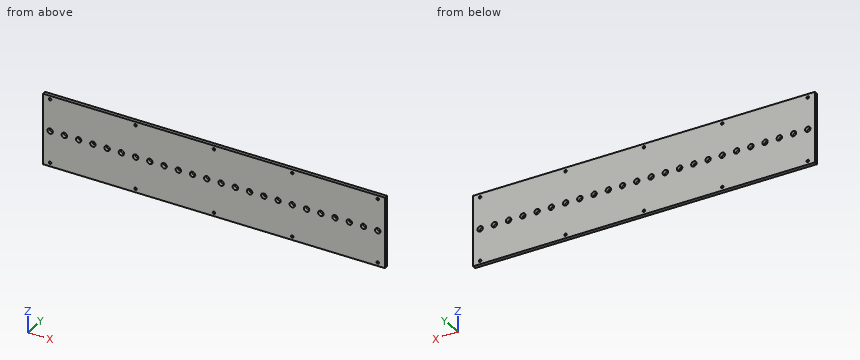
from build123d import *

# Parameters (mm, degrees)
SKETCH2_W           = 609.6
SKETCH2_H           = 127
SKETCH2_R           = 4.826
BOSS_EXTRUDE1_DEPTH = 6.35
SKETCH3_R           = 2.1828125
CUT_EXTRUDE1_DEPTH  = 6.35


with BuildPart() as part:
    # Sketch2 → Boss-Extrude1 (new body)
    with BuildSketch(Plane(origin=(0, 0, 0), x_dir=(1, 0, 0), z_dir=(0, 1, 0))):
        with Locations((304.8, 63.5)):
            Rectangle(SKETCH2_W, SKETCH2_H)
        with Locations(Location((12.7, 63.5, 0), (0, 0, 270))):
            Circle(SKETCH2_R, mode=Mode.SUBTRACT)
        with Locations(Location((38.1, 63.5, 0), (0, 0, 270))):
            Circle(SKETCH2_R, mode=Mode.SUBTRACT)
        with Locations(Location((63.5, 63.5, 0), (0, 0, 270))):
            Circle(SKETCH2_R, mode=Mode.SUBTRACT)
        with Locations(Location((88.9, 63.5, 0), (0, 0, 270))):
            Circle(SKETCH2_R, mode=Mode.SUBTRACT)
        with Locations(Location((114.3, 63.5, 0), (0, 0, 270))):
            Circle(SKETCH2_R, mode=Mode.SUBTRACT)
        with Locations(Location((139.7, 63.5, 0), (0, 0, 270))):
            Circle(SKETCH2_R, mode=Mode.SUBTRACT)
        with Locations(Location((165.1, 63.5, 0), (0, 0, 270))):
            Circle(SKETCH2_R, mode=Mode.SUBTRACT)
        with Locations(Location((190.5, 63.5, 0), (0, 0, 270))):
            Circle(SKETCH2_R, mode=Mode.SUBTRACT)
        with Locations(Location((215.9, 63.5, 0), (0, 0, 270))):
            Circle(SKETCH2_R, mode=Mode.SUBTRACT)
        with Locations(Location((241.3, 63.5, 0), (0, 0, 270))):
            Circle(SKETCH2_R, mode=Mode.SUBTRACT)
        with Locations(Location((266.7, 63.5, 0), (0, 0, 270))):
            Circle(SKETCH2_R, mode=Mode.SUBTRACT)
        with Locations(Location((292.1, 63.5, 0), (0, 0, 270))):
            Circle(SKETCH2_R, mode=Mode.SUBTRACT)
        with Locations(Location((317.5, 63.5, 0), (0, 0, 270))):
            Circle(SKETCH2_R, mode=Mode.SUBTRACT)
        with Locations(Location((342.9, 63.5, 0), (0, 0, 270))):
            Circle(SKETCH2_R, mode=Mode.SUBTRACT)
        with Locations(Location((368.3, 63.5, 0), (0, 0, 270))):
            Circle(SKETCH2_R, mode=Mode.SUBTRACT)
        with Locations(Location((393.7, 63.5, 0), (0, 0, 270))):
            Circle(SKETCH2_R, mode=Mode.SUBTRACT)
        with Locations(Location((419.1, 63.5, 0), (0, 0, 270))):
            Circle(SKETCH2_R, mode=Mode.SUBTRACT)
        with Locations(Location((444.5, 63.5, 0), (0, 0, 270))):
            Circle(SKETCH2_R, mode=Mode.SUBTRACT)
        with Locations(Location((469.9, 63.5, 0), (0, 0, 270))):
            Circle(SKETCH2_R, mode=Mode.SUBTRACT)
        with Locations(Location((495.3, 63.5, 0), (0, 0, 270))):
            Circle(SKETCH2_R, mode=Mode.SUBTRACT)
        with Locations(Location((520.7, 63.5, 0), (0, 0, 270))):
            Circle(SKETCH2_R, mode=Mode.SUBTRACT)
        with Locations(Location((546.1, 63.5, 0), (0, 0, 270))):
            Circle(SKETCH2_R, mode=Mode.SUBTRACT)
        with Locations(Location((571.5, 63.5, 0), (0, 0, 270))):
            Circle(SKETCH2_R, mode=Mode.SUBTRACT)
        with Locations(Location((596.9, 63.5, 0), (0, 0, 270))):
            Circle(SKETCH2_R, mode=Mode.SUBTRACT)
    extrude(amount=BOSS_EXTRUDE1_DEPTH)

    # Sketch3 → Cut-Extrude1 (cut)
    with BuildSketch(Plane(origin=(0, 6.35, 0), x_dir=(1, 0, 0), z_dir=(0, 1, 0))):
        with Locations(Location((12.7, 120.65, 0), (0, 0, 270))):
            Circle(SKETCH3_R)
        with Locations(Location((165.1, 120.65, 0), (0, 0, 270))):
            Circle(SKETCH3_R)
        with Locations(Location((304.8, 120.65, 0), (0, 0, 270))):
            Circle(SKETCH3_R)
        with Locations(Location((444.5, 120.65, 0), (0, 0, 270))):
            Circle(SKETCH3_R)
        with Locations(Location((596.9, 120.65, 0), (0, 0, 270))):
            Circle(SKETCH3_R)
        with Locations(Location((596.9, 6.35, 0), (0, 0, 270))):
            Circle(SKETCH3_R)
        with Locations(Location((444.5, 6.35, 0), (0, 0, 270))):
            Circle(SKETCH3_R)
        with Locations(Location((304.8, 6.35, 0), (0, 0, 270))):
            Circle(SKETCH3_R)
        with Locations(Location((165.1, 6.35, 0), (0, 0, 270))):
            Circle(SKETCH3_R)
        with Locations(Location((12.7, 6.35, 0), (0, 0, 270))):
            Circle(SKETCH3_R)
    extrude(amount=-CUT_EXTRUDE1_DEPTH, mode=Mode.SUBTRACT)


solid = part.part
Part model, mm, in its own coordinate system. Give positions to 0.01 mm unless a question says otherwise; leave off trailing zeros. Write each question's results on one line, items separated by ' | '. Start each with the question number.
Q1. Wall check: L1, parallel to Z at x = 445, y = 3.75; L2, parallel to X at y = 4.75, z = -6.35; L3, parallel to Z at x = 39, y = 5.5. Give the ranges that are in metal, low to high.
Q2. Band-saw the part on A-A on y = 1.5. Count the separate pieces of the cut face and the enclosed holes in it, plus the area to 3 significant figures.
Q3. Pin check, flat tip, straight feed: P1, Ø7.5, axis at x = 190.5, z = -63.5, coming from the +Y side. Stop position of the tip, or through.
Results are:
1) L1: z = -127 to -122.77, -118.53 to -68.3, -58.7 to -8.47, -4.23 to 0 | L2: x = 0 to 10.52, 14.88 to 162.92, 167.28 to 302.62, 306.98 to 442.32, 446.68 to 594.72, 599.08 to 609.6 | L3: z = -127 to -68.24, -58.76 to 0
2) separate pieces: 1 | enclosed holes: 34 | area: 75,500 mm²
3) P1: passes through
